from build123d import *

# Parameters (mm, degrees)
SKETCH1_R               = 37.5
SKETCH1_R_2             = 35.5
BOSS_EXTRUDE1_DEPTH     = 352.5
CUT_EXTRUDE1_REACH      = 364.336
CUT_EXTRUDE1_END_RADIUS = 35.5
SKETCH2_R               = 2.5
CIRPATTERN1_COUNT       = 6


with BuildPart() as part:
    # Sketch1 → Boss-Extrude1 (new, symmetric)
    with BuildSketch(Plane.XY):
        Circle(SKETCH1_R)
        Circle(SKETCH1_R_2, mode=Mode.SUBTRACT)
    extrude(amount=BOSS_EXTRUDE1_DEPTH, both=True)

    # Cut-Extrude1: up to this cylinder (the profile starts outside it)
    cut_extrude1_end = Plane(origin=(0, 0, 347.5), z_dir=(0, 0, -1)) * Cylinder(CUT_EXTRUDE1_END_RADIUS, 800.672, mode=Mode.PRIVATE)
    # Sketch2 → Cut-Extrude1 (cut, up to the surface)
    with BuildSketch(Plane(origin=(37.5, 0, 0), x_dir=(0, 0, -1), z_dir=(1, 0, 0)), mode=Mode.PRIVATE) as cut_extrude1_sk1:
        with Locations((-347.5, 0)):
            Circle(SKETCH2_R)
    cut_extrude1_tool1 = extrude(cut_extrude1_sk1.sketch, amount=-CUT_EXTRUDE1_REACH, mode=Mode.PRIVATE) - cut_extrude1_end
    cut_extrude1 = cut_extrude1_tool1.solids().sort_by_distance((37.5, 0, 347.5))[0]
    add(cut_extrude1, mode=Mode.SUBTRACT)

    # CirPattern1: Cut-Extrude1 ×6 about axis
    cirpattern1_axis = Axis((0, 0, 352.5), (0, 0, 1))
    for i in range(1, CIRPATTERN1_COUNT):
        add(cut_extrude1.rotate(cirpattern1_axis, i * 360 / CIRPATTERN1_COUNT), mode=Mode.SUBTRACT)


solid = part.part
The model under review builds one solid part; all positions refer to its coordinate system, in mm. Round coordinates to 2 decimals unless told otherwise and drop trailing zeros. Write each loop counter-clockwise with the first axis right and the second up, starting at its lowest first coordinate (ties: lowest second). Pieces come first, ordered by that corner, then holes. Notation, with made-up numbers: (68.25, -15) - (96.25, -15) arc R22 cw to (96.25, -8) - close; hole circle Ø8 at (88, 68.25). An arc over 180 degrees is marked (long way). One line per item, written item: value. Start each with the question number.
1. Clearance check with flat-ended pins moving along their axes: P1, Ø6, axis at y = 6, z = -18, coming from the -X side; P2, Ø2, axis at x = 25.5, z = 183.5, coming from the -Y side; P3, Ø5, axis at x = 10, z = -86, coming from the +Y side; P4, Ø4, axis at y = 0, z = 347.5, coming from the -X side. State where each tip first meets the part, or that it passes through.
2. Consider section B-B on y = -14.5. Write out the cut boundary in (x, z), and give its area (3 significant figures).
3. The part is to be moulded in two halves that separate along X. For faces 1 (the face through (33, -14, 352.5)), 2 (the face through (-7.696, -34.656, -4.935)), 3 (the face through (-4.88, 37.18, 4.94)), say which applies: released by +X, released by -X, zero draft, split by the parting line, or undercut.
4. To check wall thickness, follow L1, parallel to X at y = 0.5, z = -82; L2, parallel to X at y = -2, z = 266. State the ranges of each line that lie inside material, in increasing order. Write a range as from..to.
5. Consider section A-A on x = 0. Write out the cut boundary in (y, z), and give its area (3 significant figures).
6. Consider section C-C on z = -16. Write out the cut boundary in (x, y), and give its area (3 significant figures).
Checks:
1. P1: stops at x = -37.38
1. P2: stops at y = -28.39
1. P3: stops at y = 36.74
1. P4: passes through
2. outline: (-34.58, -352.5) - (-32.4, -352.5) - (-32.4, 352.5) - (-34.58, 352.5) - close; (32.4, -352.5) - (34.58, -352.5) - (34.58, 352.5) - (32.4, 352.5) - close
2. area: 3,070 mm^2
3. face 1: zero draft
3. face 2: undercut
3. face 3: split by the parting line
4. L1: x = -37.5..-35.5, 35.5..37.5
4. L2: x = -37.45..-35.44, 35.44..37.45
5. outline: (-37.5, -352.5) - (-35.5, -352.5) - (-35.5, 352.5) - (-37.5, 352.5) - close; (35.5, -352.5) - (37.5, -352.5) - (37.5, 352.5) - (35.5, 352.5) - close
5. area: 2,820 mm^2
6. outline: circle Ø75 at (0, 0); hole circle Ø71 at (0, 0)
6. area: 459 mm^2
